Part model, mm, in its own coordinate system. A direction names the side the tool comes from. Round coordinates to 2 decimals unless told otherwise and drop trailing zeros. Order: outer loops, then holes, each group sorted by start corner. A loop starts at its lowest first (then second) coordinate and runs counter-clockwise, first axis right, second up. Notation, with made-up numbers: (-12, 68.25) - (22, 68.25) arc R29 cw to (22, 97.25) - close; hole circle Ø6 at (29.5, 77). An arc over 180 degrees is marked (long way). Return JSON: item names as keys, results as strings. Group by question number.
Item 1: Tool access for faces 5 (the face through (-25.052, -2, 21)), 6 (the face through (17.748, -2, 69)): list every direction of +Z, -Z, +X, -X, +Y, -Y with a clear straight run to the whole face (end or side of a thin tool).
Item 2: Drop flat-ended pins along their axis: pin 1 (1.6 mm diameter, centred on x = 15.5, y = -2, fed in from +Z); pin 2 (3.5 mm diameter, centred on x = 11.95, z = -22.07, fed in from +Y); pin 3 (1.6 mm diameter, centred on y = -2.5, z = 70.5, fed in from +X); pin 4 (1 mm diameter, centred on x = 15.5, y = -1.5, fed in from -Z). Give the stop position or say it passes through.
Item 3: Saw through at A-A on z = 71.5. List the corners of the cut face in (x, y).
Item 4: Saw through at C-C on y = -2.7. List the corners of the cut face in (x, z), and give its area (3 significant figures).
Item 5: Saw through at D-D on x = -15.5. List the corners of the cut face in (y, z), and give its area (3 significant figures).
Item 6: Saw through at B-B on x = 0. List the corners of the cut face in (y, z), and give its area (3 significant figures).
Item 7: Two-plate mould, pull along X, no slides. Class faces 1 (the face through (24.948, -2, 20)), 2 (the face through (0.5, -1.58, 87.92)), 3 (the face through (16, -2, 62.927)), 4 (the face through (-4.16, -1.578, 42.115)): released by +X, released by -X, zero draft, split by the parting line, or undercut.
Item 8: Probe probe 1 along X at (y, z) = (-0.15, -23); probe 2 along Z at (x, y) = (16, -0.55); probe 3 along Z at (x, y) = (12.5, -0.35). List the from-to ranges inside material, lowest first.
```python
from build123d import *

# Parameters (mm, degrees)
F0_R     = 1.6
F0_W     = 3.4
F0_H     = 12.5
F1_DEPTH = 3.2


with BuildPart() as f1:
    # F0 (on Front) → F1 (new body)
    with BuildSketch(Plane.XZ):
        with BuildLine():
            Line((-25.051908, 62.927413), (-25.051908, -22.072587))
            ThreePointArc((-25.051908, -22.072587), (-0.051908, -47.072587), (24.948092, -22.072587))
            Line((24.948092, -22.072587), (24.948092, 62.927413))
            ThreePointArc((24.948092, 62.927413), (-0.051908, 87.927413), (-25.051908, 62.927413))
        make_face()
        with Locations((-0.051908, -22.072587)):
            Circle(F0_R, mode=Mode.SUBTRACT)
        with Locations((11.948092, -22.072587)):
            Circle(F0_R, mode=Mode.SUBTRACT)
        with Locations((-3.952201, 40.528232)):
            Circle(F0_R, mode=Mode.SUBTRACT)
        with Locations((16.048092, 69.17741)):
            Rectangle(F0_W, F0_H, mode=Mode.SUBTRACT)
    extrude(amount=F1_DEPTH)


solid = f1.part
```
Filled in:
{
 "1": {"face 5": "+Z, -Z, -X, +Y, -Y", "face 6": "+Y, -Y"},
 "2": {"pin 1": "stops at z = 83.11", "pin 2": "stops at y = 0", "pin 3": "stops at x = 24.01", "pin 4": "stops at z = -42.03"},
 "3": {"outline": "(-23.54, -3.2) - (14.35, -3.2) - (14.35, 0) - (-23.54, 0) - close; (17.75, -3.2) - (23.43, -3.2) - (23.43, 0) - (17.75, 0) - close"},
 "4": {"outline": "(-25.05, -22.07) arc R25 ccw to (24.95, -22.07) - (24.95, 62.93) arc R25 ccw to (-25.05, 62.93) - close; hole circle Ø3.2 at (-3.95, 40.53); hole circle Ø3.2 at (-0.05, -22.07); hole circle Ø3.2 at (11.95, -22.07); hole (14.35, 62.93) - (17.75, 62.93) - (17.75, 75.43) - (14.35, 75.43) - close", "area": "6,150 mm^2"},
 "5": {"outline": "(-3.2, -41.73) - (0, -41.73) - (0, 82.58) - (-3.2, 82.58) - close", "area": "398 mm^2"},
 "6": {"outline": "(-3.2, -47.07) - (0, -47.07) - (0, -23.67) - (-3.2, -23.67) - close; (-3.2, -20.47) - (0, -20.47) - (0, 87.93) - (-3.2, 87.93) - close", "area": "422 mm^2"},
 "7": {"face 1": "released by +X", "face 2": "split by the parting line", "face 3": "undercut", "face 4": "undercut"},
 "8": {"probe 1": "x = -25.03 to -1.36, 1.25 to 10.64, 13.25 to 24.93", "probe 2": "z = -41.24 to 62.93, 75.43 to 82.09", "probe 3": "z = -43.69 to -23.57, -20.57 to 84.55"}
}
